```python
from build123d import *

# Parameters (mm, degrees)
F0_W     = 76.2
F0_H     = 63.5
F1_DEPTH = 15.24
F2_R     = 17.535676
F3_DEPTH = 15.241
F4_W     = 76.2
F4_H     = 20.012378
F5_DEPTH = 30.48
F6_W     = 20.0152
F6_H     = 20.012378
F7_DEPTH = 15.24


with BuildPart() as f1:
    # F0 (on Top) → F1 (new body)
    with BuildSketch(Plane.XY):
        with BuildLine():
            Line((-38.1, 31.75), (38.1, 31.75))
            ThreePointArc((38.1, 31.75), (0, 69.85), (-38.1, 31.75))
        make_face()
        Rectangle(F0_W, F0_H)
    extrude(amount=F1_DEPTH)

    # F2 (on face) → F3 (cut, through all)
    with BuildSketch(Plane.XY.offset(15.24)):
        with Locations((0, 31.75)):
            Circle(F2_R)
    extrude(amount=-F3_DEPTH, mode=Mode.SUBTRACT)

    # F4 (on face) → F5 (join)
    with BuildSketch(Plane.XY.offset(15.24)):
        with Locations((0, -21.743811)):
            Rectangle(F4_W, F4_H)
    extrude(amount=F5_DEPTH)

    # F6 (on face) → F7 (cut)
    with BuildSketch(Plane.XY.offset(45.72)):
        with Locations((28.0924, -21.743811)):
            Rectangle(F6_W, F6_H)
    extrude(amount=-F7_DEPTH, mode=Mode.SUBTRACT)


solid = f1.part
```
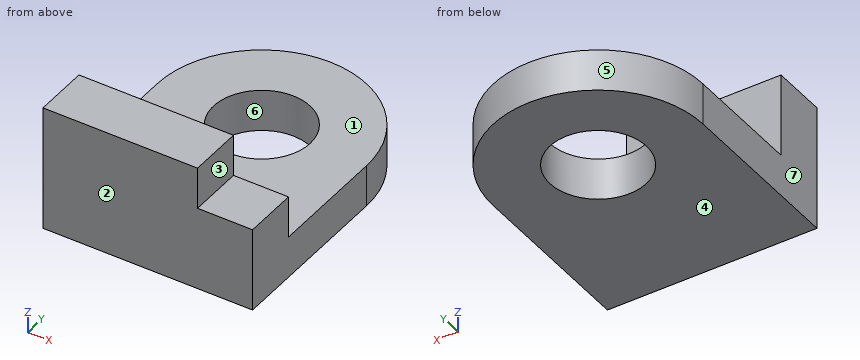
Can you work these out from the model? Positions are in its coordinate system, mm. Face numbers are marked on the shaded views. A direction names the side the tool comes from. Coordinates: 2 decimals unless noted, no trailing zeros. Write each loop counter-clockwise with the first axis right and the second up, starting at its lowest first coordinate (ties: lowest second). Pieces come first, ordered by that corner, then holes. Notation, with made-up numbers: M 75,-28.5 L 134,-28.5 A26 ccw 134,6.5 Z; hole C -20.5,24.5 d9. An arc over 180 degrees is marked long. Write item = value, one per line. Start each with the question number.
Q1. If I drill on L1, parallel to X at y = 31, z = 3; L2, parallel to Y at x = 0, z = 3; L3, parallel to Z at x = 24.5, y = 46.5, over which ranges is the centre line in solid material (lowest first)? Write a range as [from, to].
Q2. I'm going to push flat-ended pins straight in: pin 1 (8 mm diameter, centred on y = 44, z = 12, fed in from +X); pin 2 (1.5 mm diameter, centred on y = -21.5, z = 36, fed in from +X); pin 3 (8 mm diameter, centred on x = -17.5, z = 15, fed in from +Y); pin 4 (12 mm diameter, centred on y = -19, z = 36, fed in from +X). Where does each tip first touch, or does it pass through?
Q3. If we section it at B-B, the plane y = 45.5: Write out the boundary of the cut face in (x, z).
Q4. Thinking about a two-plate mould opening in X: for the marked faces 4, 5, 6 and 7, which applies, released by +X, released by -X, zero draft, split by the parting line, or undercut?
Q5. On a 3-axis mill with a long thin cutter (end or side, diameter ignored), from which of +Z, -Z, +X, -X, +Y, -Y can I reach the whole of each face in a straight line? I mean the marked faces 1, 2 and 3. Say none if no direction works.
Q6. If we section it at C-C, the plane z = 5.5: Write out the boundary of the cut face in (x, y).
Q7. If we section it at D-D, the plane y = -20: Write out the boundary of the cut face in (x, z).
Q8. If we section it at A-A, the plane x = 0: Write out the boundary of the cut face in (y, z).
Check sheet entries:
q1.L1 = [-38.1, -17.52], [17.52, 38.1]
q1.L2 = [-31.75, 14.21], [49.29, 69.85]
q1.L3 = [0, 15.24]
q2.pin_1 = 37.2
q2.pin_2 = 18.08
q2.pin_3 = 67.38
q2.pin_4 = 38.1
q3.outline = M -35.53,0 L -10.88,0 L -10.88,15.24 L -35.53,15.24 Z; M 10.88,0 L 35.53,0 L 35.53,15.24 L 10.88,15.24 Z
q4.face_4 = zero draft
q4.face_5 = split by the parting line
q4.face_6 = undercut
q4.face_7 = released by -X
q5.face_1 = +Z, +X, -X, +Y
q5.face_2 = +Z, -Z, +X, -X, -Y
q5.face_3 = +Z, +X, +Y, -Y
q6.outline = M -38.1,-31.75 L 38.1,-31.75 L 38.1,31.75 A38.1 ccw -38.1,31.75 Z; hole C 0,31.75 d35.07
q7.outline = M -38.1,0 L 38.1,0 L 38.1,30.48 L 18.08,30.48 L 18.08,45.72 L -38.1,45.72 Z
q8.outline = M -31.75,0 L 14.21,0 L 14.21,15.24 L -11.74,15.24 L -11.74,45.72 L -31.75,45.72 Z; M 49.29,0 L 69.85,0 L 69.85,15.24 L 49.29,15.24 Z
